```python
from build123d import *

# Parameters (mm, degrees)
SKETCH2_W                                            = 33.3756
SKETCH2_H                                            = 76.48702
BODY_EXTRUDE_DEPTH                                   = 3.175
ROUND_EXTRUDE_DEPTH                                  = 6.35
SKETCH5_W                                            = 20.6756
SKETCH5_H                                            = 35.3314
RECTANGLE_CUT_DEPTH                                  = 88.03940876
BACK_EDGE_FILLET_R                                   = 12.7
OUTER_FILLET_R                                       = 9.525
INNER_FILLET_R                                       = 7.9375
CSK_FOR_M8_CROSS_COUNTERSUNK_HEAD_SCREW1_D           = 8
CSK_FOR_M8_CROSS_COUNTERSUNK_HEAD_SCREW1_DEPTH       = 33.782
CSK_FOR_M8_CROSS_COUNTERSUNK_HEAD_SCREW1_CSINK_D     = 16
CSK_FOR_M8_CROSS_COUNTERSUNK_HEAD_SCREW1_CSINK_ANGLE = 90
VERTICAL_HOLES_DEPTH                                 = 87.191021329
VERTICAL_HOLES_DEPTH_BACK                            = 87.191021329
SKETCH9_R                                            = 4.9022


with BuildPart() as part:
    # Sketch2 → Body Extrude (new, symmetric)
    with BuildSketch(Plane(origin=(0, 0, 0), x_dir=(0, 0, -1), z_dir=(1, 0, 0))):
        with Locations((16.6878, 38.24351)):
            Rectangle(SKETCH2_W, SKETCH2_H)
    extrude(amount=BODY_EXTRUDE_DEPTH, both=True)

    # Sketch3 → Round Extrude (add)
    with BuildSketch(Plane.XY):
        with BuildLine():
            Line((18.936083517, 44.59351), (18.936083517, 31.89351))
            ThreePointArc((18.936083517, 31.89351), (16.776632986, 27.073011115), (13.511311574, 22.921130557))
            ThreePointArc((13.511311574, 22.921130557), (11.564427885, 21.602067983), (9.271, 21.082))
            ThreePointArc((9.271, 21.082), (4.758252665, 18.954997631), (3.175, 14.224))
            Line((3.175, 14.224), (-3.175, 6.35))
            ThreePointArc((-3.175, 6.35), (-15.275957763, 17.02760796), (-21.556837243, 31.89351))
            Line((-21.556837243, 31.89351), (-21.556837243, 44.59351))
            ThreePointArc((-21.556837243, 44.59351), (-15.275957763, 59.45941204), (-3.175, 70.13702))
            Line((-3.175, 70.13702), (3.175, 62.26302))
            ThreePointArc((3.175, 62.26302), (4.758252665, 57.532022369), (9.271, 55.40502))
            ThreePointArc((9.271, 55.40502), (11.564427885, 54.884952017), (13.511311574, 53.565889443))
            ThreePointArc((13.511311574, 53.565889443), (16.776632986, 49.414008885), (18.936083517, 44.59351))
        make_face()
    round_extrude = extrude(amount=-ROUND_EXTRUDE_DEPTH)

    # Round Extrude Mirrored: Round Extrude across plane
    add(round_extrude.mirror(Plane(origin=(0, 0, -16.6878), x_dir=(1, 0, 0), z_dir=(0, 0, -1))))

    # Sketch5 → Rectangle Cut (cut, through all)
    with BuildSketch(Plane(origin=(3.175, 0, 0), x_dir=(0, 0, -1), z_dir=(1, 0, 0))):
        with Locations((16.6878, 38.24351)):
            Rectangle(SKETCH5_W, SKETCH5_H)
    extrude(amount=-RECTANGLE_CUT_DEPTH, mode=Mode.SUBTRACT)

    # Back Edge Fillet
    # the kernel refuses this fillet: 12.7 mm, written as the material it adds along each edge
    with BuildSketch(Plane(origin=(-3.175, 6.35, -33.3756), x_dir=(-0.8366334248395991, 0.5477631901115323, 0), z_dir=(0, 0, 1)), Plane(origin=(-3.175, 70.13702, 0), x_dir=(-0.8366334248396001, -0.5477631901115311, 0), z_dir=(0, 0, -1))) as back_edge_fillet_piece_1:
        with BuildLine():
            CenterArc((6.881526007, 12.658647204), BACK_EDGE_FILLET_R, 215.339993456, 50.03506631)
            Line((-3.478296257, 5.312622248), (-3.685492702, 5.165701749))
            ThreePointArc((-3.685492702, 5.165701749), (-1.951653019, 2.517179274), (-0.21250489, -0.13913185))
            Line((-0.21250489, -0.13913185), (0.020480732, -0.253172944))
            ThreePointArc((0.020480732, -0.253172944), (2.928744699, -0.135731002), (5.837008667, -0.253172944))
            Line((5.837008667, -0.253172944), (5.857489399, 0))
        make_face()
    extrude(amount=6.35)
    with BuildSketch(Plane(origin=(-3.175, 6.35, 0), x_dir=(-0.8366334248395991, 0.5477631901115323, 0), z_dir=(0, 0, -1)), Plane(origin=(-3.175, 70.13702, -33.3756), x_dir=(-0.8366334248396001, -0.5477631901115311, 0), z_dir=(0, 0, 1))) as back_edge_fillet_piece_2:
        with BuildLine():
            CenterArc((6.881526007, -12.658647204), BACK_EDGE_FILLET_R, 94.624940234, 50.03506631)
            Line((-3.478296257, -5.312622248), (-3.685492702, -5.165701749))
            ThreePointArc((-3.685492702, -5.165701749), (-1.951653019, -2.517179274), (-0.21250489, 0.13913185))
            Line((-0.21250489, 0.13913185), (0.020480732, 0.253172944))
            ThreePointArc((0.020480732, 0.253172944), (2.928744699, 0.135731002), (5.837008667, 0.253172944))
            Line((5.837008667, 0.253172944), (5.857489399, 0))
        make_face()
    extrude(amount=6.35)

    # Outer Fillet
    # the kernel refuses this fillet: 9.525 mm, written as the material it takes off along each edge
    with BuildSketch(Plane(origin=(26.9875, 76.48702, 0), x_dir=(0, 0, -1), z_dir=(-1, 0, 0)), Plane(origin=(-26.9875, 76.48702, -33.3756), x_dir=(0, 0, 1), z_dir=(1, 0, 0)), Plane(origin=(-26.9875, 0, -33.3756), x_dir=(0, 1, 0), z_dir=(1, 0, 0)), Plane(origin=(26.9875, 0, 0), x_dir=(0, 1, 0), z_dir=(-1, 0, 0))) as outer_fillet_piece_1:
        with BuildLine():
            CenterArc((OUTER_FILLET_R, OUTER_FILLET_R), OUTER_FILLET_R, 180, 90)
            Line((0, OUTER_FILLET_R), (0, 0))
            Line((0, 0), (OUTER_FILLET_R, 0))
        make_face()
    extrude(amount=53.975, mode=Mode.SUBTRACT)

    # Inner Fillet
    inner_fillet_edges = [part.edges().sort_by_distance(p)[0] for p in [
        (0, 55.90921, -27.0256),
        (0, 20.57781, -6.35),
        (0, 55.90921, -6.35),
        (0, 20.57781, -27.0256),
    ]]
    fillet(inner_fillet_edges, radius=INNER_FILLET_R)

    # CSK for M8 Cross Countersunk Head Screw1
    with Locations(Plane.ZY.offset(3.175)):
        with Locations((-16.6878, 66.20002), (-16.6878, 10.287)):
            CounterSinkHole(CSK_FOR_M8_CROSS_COUNTERSUNK_HEAD_SCREW1_D / 2, CSK_FOR_M8_CROSS_COUNTERSUNK_HEAD_SCREW1_CSINK_D / 2, depth=CSK_FOR_M8_CROSS_COUNTERSUNK_HEAD_SCREW1_DEPTH, counter_sink_angle=CSK_FOR_M8_CROSS_COUNTERSUNK_HEAD_SCREW1_CSINK_ANGLE)

    # Sketch9 → Vertical Holes (cut, two sides: drawn at the far end of the back side and taken through both)
    with BuildSketch(Plane.XY.offset(-VERTICAL_HOLES_DEPTH_BACK)):
        with Locations((0, 38.24351)):
            Circle(SKETCH9_R)
    extrude(amount=VERTICAL_HOLES_DEPTH + VERTICAL_HOLES_DEPTH_BACK, mode=Mode.SUBTRACT)


solid = part.part
```
For this review, take the finished solid that the model builds, in its own axes (mm). A direction names the side the tool comes from. Coordinates: 2 decimals unless noted, no trailing zeros. Write each loop counter-clockwise with the first axis right and the second up, starting at its lowest first coordinate (ties: lowest second). Pieces come first, ordered by that corner, then holes. Notation, with made-up numbers: (-19.5, 5.5) -> (-15.5, 5.5) arc R17 cw to (-15.5, 26.5) -> close; hole circle Ø10 at (59.25, 68). An arc over 180 degrees is marked (long way). Put each result on its own line as item: value.
Q1. The part is to be moulded in two halves that separate along Z. For faces 4 (the flat face through (-3.175, 14.5, -9.7)), 5 (the flat face through (0, 55.909, -17)), 6 (the cylindrical face through (-16.79, 19.31, -3.13)), 7 (the cylindrical face through (-0.02, 73.62, -30.66)), say which applies: +Z half, -Z half, draft (parallel to the pull), parting line (faces both ways), or undercut.
From the geometry:
face 4: undercut
face 5: undercut
face 6: draft
face 7: -Z half
Q2. Clearance check with flat-ended pins moving along their axes: pin 1 Ø9 at (y, z) = (66.2, -16.69) entering from -X; pin 2 Ø10 at (x, y) = (3.5, 60.5) entering from -Z; pin 3 Ø10.5 at (y, z) = (18, -20.5) entering from -X (3 decimals); pin 4 Ø14.5 at (y, z) = (13.5, -22) entering from +X. State where each tip first meets the part, or that it passes through.
From the geometry:
pin 1: stops at x = 0.32
pin 2: stops at z = -33.38
pin 3: stops at x = -3.175
pin 4: stops at x = 4.56
Q3. Take a section at C-C, the plane x = -6. State the section outline as (y, z) points (3 decimals).
From the geometry:
outline: (7.525, -33.163) arc R9.525 ccw to (9.525, -33.376) -> (66.962, -33.376) arc R9.525 ccw to (68.962, -33.163) -> (68.962, -27.026) -> (7.525, -27.026) -> close; (7.525, -6.35) -> (68.962, -6.35) -> (68.962, -0.212) arc R9.525 ccw to (66.962, 0) -> (9.525, 0) arc R9.525 ccw to (7.525, -0.212) -> close
Q4. Take a section at A-A, the plane x = 2. Count the separate pieces of the cut face and the enclosed holes in it, then the cut area to 3 significant figures.
From the geometry:
separate pieces: 2
enclosed holes: 2
area: 1,580 mm2
Q5. Tool access review of faces 1 (the flat face through (3.175, 69, -20)), 2 (the flat face through (0, 20.578, -17)), 3 (the cylindrical face through (16.815, 27.137, -30.245)): name each direction out of +Z, -Z, +X, -X, +Y, -Y from which nothing blocks a thin tool from reaching the whole face with its end or side.
From the geometry:
face 1: +X, +Y
face 2: +X, -X
face 3: +Z, -Z, +X, -Y
Q6. Take a section at D-D, the plane y = 36.5. State the section outline as (x, z) points.
From the geometry:
outline: (-21.56, -33.38) -> (-4.58, -33.38) -> (-4.58, -27.03) -> (-21.56, -27.03) -> close; (-21.56, -6.35) -> (-4.58, -6.35) -> (-4.58, 0) -> (-21.56, 0) -> close; (4.58, -33.38) -> (18.94, -33.38) -> (18.94, -27.03) -> (4.58, -27.03) -> close; (4.58, -6.35) -> (18.94, -6.35) -> (18.94, 0) -> (4.58, 0) -> close
Q7. Wall thickness on L1, parallel to Z at x = 9.5, y = 21.5; L2, parallel to Y at x = 0, z = -29.25: over which ranges is each line inside the solid? List them lowest first.
From the geometry:
L1: z = -33.38 to -27.03, -6.35 to 0
L2: y = 1.68 to 33.34, 43.15 to 74.81
Q8. Take a section at B-B, the plane y = 24. State the section outline as (x, z) points (3 decimals).
From the geometry:
outline: (-19.207, -33.376) -> (14.526, -33.376) -> (14.526, -27.026) -> (3.175, -27.026) -> (3.175, -25.616) -> (-3.175, -25.616) -> (-3.175, -27.026) -> (-19.207, -27.026) -> close; (-19.207, -6.35) -> (-3.175, -6.35) -> (-3.175, -7.759) -> (3.175, -7.759) -> (3.175, -6.35) -> (14.526, -6.35) -> (14.526, 0) -> (-19.207, 0) -> close
